Autodesk Inventor part; units mm, degrees
ref_plane "YZ Plane" through (0, 0, 0) normal (1, 0, 0) x (0, 1, 0)
ref_plane "XZ Plane" through (0, 0, 0) normal (0, 1, 0) x (-1, 0, 0)
ref_plane "XY Plane" through (0, 0, 0) normal (0, 0, 1) x (1, 0, 0)
sketch "Sketch1" plane through (0, 0, 0) normal (1, 0, 0) x (0, 1, 0)
  line L0 (0, 0) -> (-3.175, 0)
  line L1 (-3.175, 0) -> (-3.175, 25.4)
  line L2 (-3.175, 25.4) -> (0, 25.4)
  line L3 (0, 25.4) -> (0, 0)
  line L4 (0, 0) -> (-25.4, 0)
  line L5 (-25.4, 0) -> (-25.4, 3.175)
  line L6 (-25.4, 3.175) -> (0, 3.175)
  line L7 (0, 3.175) -> (0, 0)
  dimension "d0" = 3.175
  dimension "d1" = 25.4
  dimension "d2" = 25.4
  dimension "d3" = 3.175
extrude "Extrusion1" add sketch "Sketch1" along normal blind 241.3
sketch "Sketch2" plane through (0, 0, 25.4) normal (0, 1, 0) x (1, 0, 0)
  line L0 (0, 25.4) -> (0, 0)
  line L1 (0, 0) -> (241.3, 0)
  line L2 (241.3, 25.4) -> (241.3, 0)
  line L3 (0, 25.4) -> (241.3, 25.4)
  point P0 (228.6, 12.7)
  point P1 (12.7, 12.7)
  dimension "d6" = 12.7
  dimension "d7" = 12.7
  dimension "d8" = 12.7
  dimension "d9" = 228.6
hole "Hole1" at (228.6, 0, 12.7) at (12.7, 0, 12.7) direction (0, -1, 0) diameter 6.7469 end through all
properties part number "front slider guard" material "Aluminum 6061"
The model under review builds one solid part; all positions refer to its coordinate system, in mm. A direction names the side the tool comes from. Give positions to 0.01 mm unless a question says otherwise; leave off trailing zeros. Order: outer loops, then holes, each group sorted by start corner. A loop starts at its lowest first (then second) coordinate and runs counter-clockwise, first axis right, second up. Notation, with made-up numbers: M 46,63 L 100,63 A14 ccw 100,86 Z; hole C 15.5,30 d10. An arc over 180 degrees is marked long. Answer in a Markdown table with one row per item. Add a question column.
1. Add section D-D on x = 201.5. State the section outline as (y, z) points (3 decimals), plus the area to 3 significant figures.
2. Add section C-C on y = -23. State the section outline as (x, z) points (3 decimals).
3. To check wall thickness, follow line 1 along X through (y, z) = (-1.1, 12.7); line 2 along Z through (x, y) = (12.7, -0.65); line 3 along Z through (x, y) = (151.5, -8.75) (3 decimals). State the ranges of each line that lie inside material, in increasing order.
4. Mouldability with a two-part tool opening along X and no side actions: class faces 1 (the flat face through (0, -7, 2)), 2 (the cylindrical face through (9.355, -1.61, 12.261)), 3 (the flat face through (241.3, -7, 2)) as released by +X, released by -X, zero draft, split by the parting line, or undercut.
5. Add section A-A on z = 12.7. State the section outline as (x, y) points (3 decimals), plus the area to 3 significant figures.
6. Machinability: for faces 4 (the flat face through (119, 0, 13)), 5 (the flat face through (119, -14, 3.175)), which of the approach directions +Z, -Z, +X, -X, +Y, -Y give a long, thin tool a straight path to every point of the face, cutting with its end or side? Answer none if there is none.
7. Add section B-B on x = 12.7. State the section outline as (y, z) points (3 decimals).
8. For pin 1 Ø6.5 at (x, y) = (159.5, -13.5) entering from +Z (3 decimals); pin 2 Ø4 at (y, z) = (-5.5, 18) entering from -X; pin 3 Ø11 at (x, z) = (84.5, 19.5) entering from -Y (3 decimals), all flat-tipped, find the tip position at first contact; note any pin that passes through.
The answers:
| question | item | result |
|---|---|---|
| 1 | outline | M -25.4,0 L 0,0 L 0,25.4 L -3.175,25.4 L -3.175,3.175 L -25.4,3.175 Z |
| 1 | area | 151 mm2 |
| 2 | outline | M 0,0 L 241.3,0 L 241.3,3.175 L 0,3.175 Z |
| 3 | line 1 | 0 to 9.33, 16.07 to 225.23, 231.97 to 241.3 |
| 3 | line 2 | 0 to 9.33, 16.07 to 25.4 |
| 3 | line 3 | 0 to 3.175 |
| 4 | face 1 | released by -X |
| 4 | face 2 | undercut |
| 4 | face 3 | released by +X |
| 5 | outline | M 0,-3.175 L 9.327,-3.175 L 9.327,0 L 0,0 Z; M 16.073,-3.175 L 225.227,-3.175 L 225.227,0 L 16.073,0 Z; M 231.973,-3.175 L 241.3,-3.175 L 241.3,0 L 231.973,0 Z |
| 5 | area | 723 mm2 |
| 6 | face 4 | +Z, -Z, +X, -X, +Y |
| 6 | face 5 | +Z, +X, -X, -Y |
| 7 | outline | M -25.4,0 L 0,0 L 0,9.327 L -3.175,9.327 L -3.175,3.175 L -25.4,3.175 Z; M -3.175,16.073 L 0,16.073 L 0,25.4 L -3.175,25.4 Z |
| 8 | pin 1 | z = 3.175 |
| 8 | pin 2 | through |
| 8 | pin 3 | y = -3.175 |
